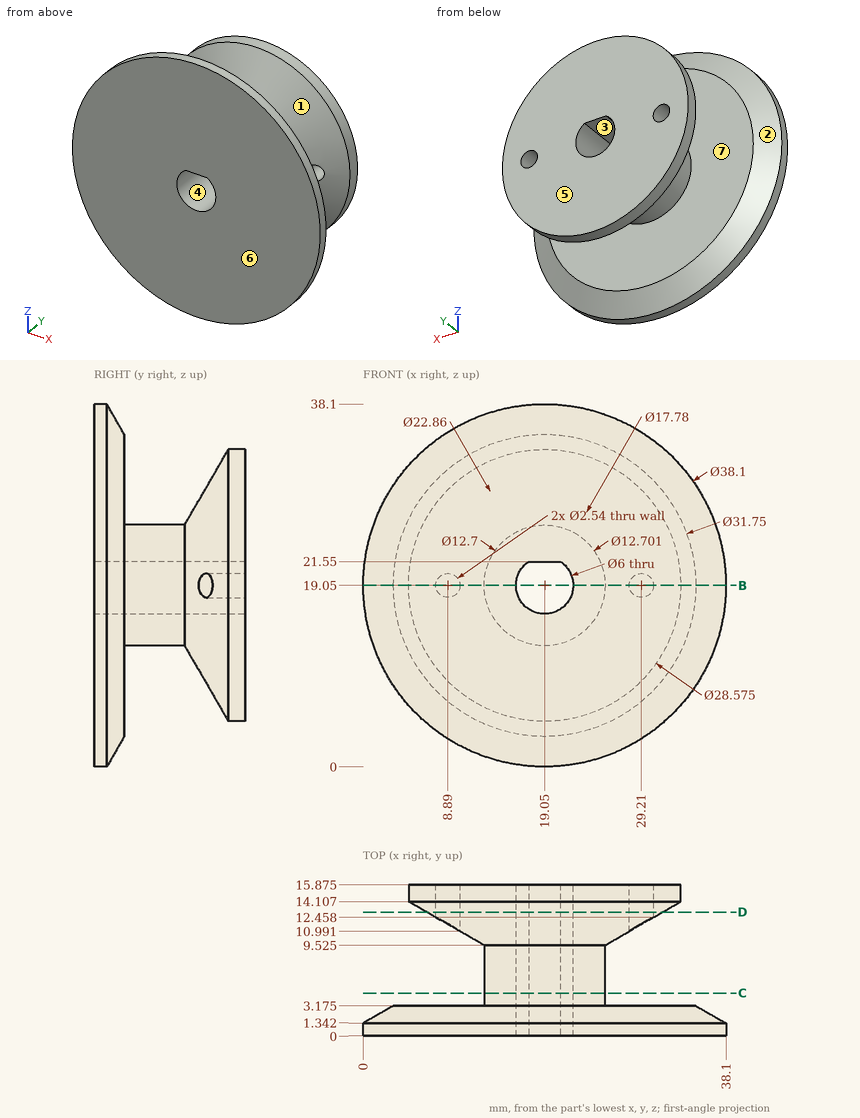
Geometry check sheet. Reference: drawing and pictorial views, mm from the part's lowest x, y, z. A direction names the side the tool comes from. Round coordinates to 2 decimals unless told otherwise and drop trailing zeros. Write each loop counter-clockwise with the first axis right and the second up, starting at its lowest first coordinate (ties: lowest second). Pieces come first, ordered by that corner, then holes. Notation, with made-up numbers: (-22.5, -17) -> (0.5, -17) arc R13 cw to (0.5, -13) -> close; hole circle Ø6 at (-38.5, 2.25). An arc over 180 degrees is marked (long way). One line per question, with ' | ' between items. Start each with the question number.
1. Release check for a two-part mould opening along Y. For the marked faces 4, 5, 6 and 7 record: +Y half, -Y half, draft (parallel to the pull), parting line (faces both ways), or undercut.
2. Scan lines: line 1 along X through (y, z) = (14.7, 19.05); line 2 along X through (y, z) = (15.25, 18) (1 decimal); line 3 along Z through (x, y) = (19.05, 6.5). Record each from-to range of solid material in increasing order. Write a range as from..to.
3. Depth check by flat-ended pin: pin 1 (3.5 mm diameter, centred on x = 19.5, y = 5.5, fed in from -Z); pin 2 (6 mm diameter, centred on y = 14, z = 20.5, fed in from -X); pin 3 (1.5 mm diameter, centred on y = 8, z = 13.5, fed in from +X). Enter the tip coordinate at first touch or a pass-through.
4. Set-up check for the marked faces 1, 2 and 3: record each of +Z, -Z, +X, -X, +Y, -Y from which the full face is reachable in a straight line by a thin tool's end or side.
5. Sectioned sample at D-D, the plane y = 13. Record the cut outline in (x, z).
6. Sectioned sample at B-B, the plane z = 19.05. Count the separate pieces of the cut face and the enclosed holes in it.
7. Sectioned sample at C-C, the plane y = 4.5. Record the cut outline in (x, z).
Taken from the geometry:
1) face 4: draft | face 5: +Y half | face 6: -Y half | face 7: undercut
2) line 1: x = 4.76..7.62, 10.16..16.05, 22.05..27.94, 30.48..33.34 | line 2: x = 4.8..8.2, 9.6..16.2, 21.9..28.5, 29.9..33.3 | line 3: z = 12.7..16.05, 21.55..25.4
3) pin 1: stops at z = 12.7 | pin 2: stops at x = 4.76 | pin 3: stops at x = 23.21
4) face 1: none | face 2: +Y | face 3: +Y, -Y
5) outline: circle Ø24.74 at (19.05, 19.05); hole circle Ø2.54 at (8.89, 19.05); hole (17.39, 21.55) arc R3 ccw (long way) to (20.71, 21.55) -> close; hole circle Ø2.54 at (29.21, 19.05)
6) separate pieces: 4 | enclosed holes: 0
7) outline: circle Ø12.7 at (19.05, 19.05); hole (17.39, 21.55) arc R3 ccw (long way) to (20.71, 21.55) -> close
